from build123d import *

# Parameters (mm, degrees)
SKETCH1_W          = 4
SKETCH1_H          = 4
KEYEXTRUSION_DEPTH = 16
ENDRADII_R         = 2


with BuildPart() as part:
    # Sketch1 → KeyExtrusion (new body)
    with BuildSketch(Plane.XY):
        with Locations((2, 2)):
            Rectangle(SKETCH1_W, SKETCH1_H)
    extrude(amount=KEYEXTRUSION_DEPTH)

    # EndRadii
    endradii_edges = [part.edges().sort_by_distance(p)[0] for p in [
        (0, 2, 0),
        (4, 2, 0),
        (0, 2, 16),
        (4, 2, 16),
    ]]
    fillet(endradii_edges, radius=ENDRADII_R - 0.0001)  # a hair under: the kernel refuses the full size


solid = part.part
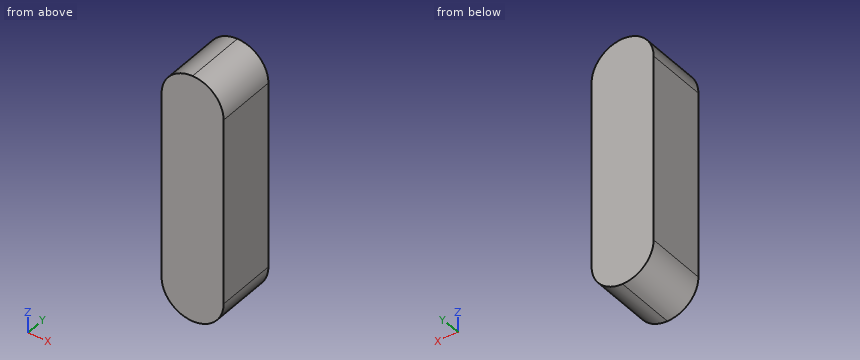
Build history of the part. All positions in model axes, mm. Give positions to 0.01 mm unless a question says otherwise; leave off trailing zeros. Loops run counter-clockwise (first coordinate to the right, second up) from the corner with the lowest first, then second, coordinate; pieces in that order, holes last. Notation, with made-up numbers: (23.5, 89) - (37.5, 89) arc R26 cw to (37.5, 107) - close; hole circle Ø2 at (9, 63). An arc over 180 degrees is marked (long way). Write item = value, one per line. Start each with the question number.
1) Band-saw the part on B-B on x = 3.45. Give the cut face in (y, z), plus the area to 3 significant figures.
2) Probe probe 1 along Z at (x, y) = (1.9, 1.7); probe 2 along Z at (x, y) = (1.05, 2.7); probe 3 along X at (y, z) = (1, 1). List the from-to ranges inside material, lowest first. Write a range as from..to.
3) Drop a flat-ended pin along its axis: pin 1 Ø1 at (x, y) = (3, 2.5) entering from -Z. Give the stop position or say it passes through.
Final values:
q1.outline = (0, 0.62) - (4, 0.62) - (4, 15.38) - (0, 15.38) - close
q1.area = 59.0 mm²
q2.probe_1 = 0..16
q2.probe_2 = 0.24..15.76
q2.probe_3 = 0.27..3.73
q3.pin_1 = 0.06
